The model under review builds one solid part; all positions refer to its coordinate system, in mm. A direction names the side the tool comes from. Give positions to 0.01 mm unless a question says otherwise; leave off trailing zeros. Order: outer loops, then holes, each group sorted by start corner. A loop starts at its lowest first (then second) coordinate and runs counter-clockwise, first axis right, second up. Notation, with made-up numbers: M 69.25,22 L 75.25,22 A19 ccw 75.25,54 Z; hole C 85.5,-0.75 d11. An arc over 180 degrees is marked long. One line per question, with ' | ' between items. Start each with the question number.
1. The part is to be moulded in two halves that separate along Y. For faces 1 (the face through (-73, 38, 0)), 2 (the face through (1, 60, 0)), 3 (the face through (-102, 1, 0)), say which applies: +Y half, -Y half, draft (parallel to the pull), parting line (faces both ways), or undercut.
2. We need section A-A on x = -76. Write out the cut boundary in (y, z), then the cut area to 4 significant figures.
3. We need section C-C on z = -1.75. Write out the cut boundary in (x, y).
4. We need section B-B on y = 34. Write out the cut boundary in (x, z).
5. Insertion check: P1, Ø4, axis at x = -96.5, y = -53, coming from the -Z side. The pin has a flat end and moves straight along its axis. Give the tip position at first contact, or say it passes through.
6. For faces 4 (the face through (-95.867, 49.095, -2.535)), 5 (the face through (75.9, 42.5, -2.5)), 6 (the face through (76, 45, 2)), 7 (the face through (-1, 1, -5)), list the 3-axis set-ups (+Z, -Z, +X, -X, +Y, -Y) from which the entire face can be reached by the end or side of a thin tool; tool diameter is ignored.
7. Wall thickness on L1, parallel to X at y = 36, z = 4; L2, parallel to Y at x = -95, z = -2.1; L3, parallel to Y at x = -95, z = 3: over which ranges is each line inside the solid? List them lowest first.
```python
from build123d import *

# Parameters (mm, degrees)
F0_R     = 4
F1_DEPTH = 5
F2_DEPTH = 5
F3_DEPTH = 5
F0_R_2   = 1.6
F4_DEPTH = 5
F5_DEPTH = 5
F6_DEPTH = 5
F7_DEPTH = 5
F8_DEPTH = 5


with BuildPart() as f1:
    # F0 (on Top) → F1 (new body)
    with BuildSketch(Plane.XY):
        Polygon((102, 53), (102, 60), (95, 60), (-95, 60), (-102, 60), (-102, 53), (-102, -53), (-102, -60), (-95, -60), (95, -60), (102, -60), (102, -53), align=None)
        with Locations((-95, -53)):
            Circle(F0_R, mode=Mode.SUBTRACT)
        with Locations((95, -53)):
            Circle(F0_R, mode=Mode.SUBTRACT)
        with BuildLine():
            ThreePointArc((-81, 40), (-76, 45), (-71, 40))
            Line((-71, 40), (-71, 27))
            ThreePointArc((-71, 27), (-76, 22), (-81, 27))
            Line((-81, 27), (-81, 40))
        make_face(mode=Mode.SUBTRACT)
        with Locations((-95, 53)):
            Circle(F0_R, mode=Mode.SUBTRACT)
        with BuildLine():
            Line((71, 27), (71, 40))
            ThreePointArc((71, 40), (76, 45), (81, 40))
            Line((81, 40), (81, 27))
            ThreePointArc((81, 27), (76, 22), (71, 27))
        make_face(mode=Mode.SUBTRACT)
        with Locations((95, 53)):
            Circle(F0_R, mode=Mode.SUBTRACT)
    extrude(amount=-F1_DEPTH)

    # F0 (on Top) → F2 (join)
    with BuildSketch(Plane.XY):
        with BuildLine():
            Line((-71, 27), (-71, 40))
            ThreePointArc((-71, 40), (-76, 45), (-81, 40))
            Line((-81, 40), (-81, 27))
            ThreePointArc((-81, 27), (-80.330127, 29.5), (-78.5, 31.330127))
            Line((-78.5, 31.330127), (-78.5, 40))
            ThreePointArc((-78.5, 40), (-76, 42.5), (-73.5, 40))
            Line((-73.5, 40), (-73.5, 31.330127))
            ThreePointArc((-73.5, 31.330127), (-71.669873, 29.5), (-71, 27))
        make_face()
    extrude(amount=-F2_DEPTH)

    # F0 (on Top) → F3 (join)
    with BuildSketch(Plane.XY):
        Polygon((102, 53), (102, 60), (95, 60), (-95, 60), (-102, 60), (-102, 53), (-102, -53), (-102, -60), (-95, -60), (95, -60), (102, -60), (102, -53), align=None)
        with Locations((-95, -53)):
            Circle(F0_R, mode=Mode.SUBTRACT)
        with Locations((95, -53)):
            Circle(F0_R, mode=Mode.SUBTRACT)
        with BuildLine():
            ThreePointArc((-81, 40), (-76, 45), (-71, 40))
            Line((-71, 40), (-71, 27))
            ThreePointArc((-71, 27), (-76, 22), (-81, 27))
            Line((-81, 27), (-81, 40))
        make_face(mode=Mode.SUBTRACT)
        with Locations((-95, 53)):
            Circle(F0_R, mode=Mode.SUBTRACT)
        with BuildLine():
            Line((71, 27), (71, 40))
            ThreePointArc((71, 40), (76, 45), (81, 40))
            Line((81, 40), (81, 27))
            ThreePointArc((81, 27), (76, 22), (71, 27))
        make_face(mode=Mode.SUBTRACT)
        with Locations((95, 53)):
            Circle(F0_R, mode=Mode.SUBTRACT)
    extrude(amount=F3_DEPTH)

    # F0 (on Top) → F4 (join)
    with BuildSketch(Plane.XY):
        with Locations((95, -53)):
            Circle(F0_R)
        with Locations((95, -53)):
            Circle(F0_R_2, mode=Mode.SUBTRACT)
    extrude(amount=F4_DEPTH)

    # F0 (on Top) → F5 (join)
    with BuildSketch(Plane.XY):
        with BuildLine():
            ThreePointArc((81, 40), (76, 45), (71, 40))
            Line((71, 40), (71, 27))
            ThreePointArc((71, 27), (71.669873, 29.5), (73.5, 31.330127))
            Line((73.5, 31.330127), (73.5, 40))
            ThreePointArc((73.5, 40), (76, 42.5), (78.5, 40))
            Line((78.5, 40), (78.5, 31.330127))
            ThreePointArc((78.5, 31.330127), (80.330127, 29.5), (81, 27))
            Line((81, 27), (81, 40))
        make_face()
    extrude(amount=-F5_DEPTH)

    # F0 (on Top) → F6 (join)
    with BuildSketch(Plane.XY):
        with Locations((95, 53)):
            Circle(F0_R)
        with Locations((95, 53)):
            Circle(F0_R_2, mode=Mode.SUBTRACT)
    extrude(amount=F6_DEPTH)

    # F0 (on Top) → F7 (join)
    with BuildSketch(Plane.XY):
        with Locations((-95, 53)):
            Circle(F0_R)
        with Locations((-95, 53)):
            Circle(F0_R_2, mode=Mode.SUBTRACT)
    extrude(amount=F7_DEPTH)

    # F0 (on Top) → F8 (join)
    with BuildSketch(Plane.XY):
        with Locations((-95, -53)):
            Circle(F0_R)
        with Locations((-95, -53)):
            Circle(F0_R_2, mode=Mode.SUBTRACT)
    extrude(amount=F8_DEPTH)


solid = f1.part
```
Entries:
1) face 1: undercut | face 2: +Y half | face 3: draft
2) outline: M -60,-5 L 22,-5 L 22,5 L -60,5 Z; M 42.5,-5 L 60,-5 L 60,5 L 45,5 L 45,0 L 42.5,0 Z | area: 982.5 mm^2
3) outline: M -102,-60 L 102,-60 L 102,60 L -102,60 Z; hole C -95,-53 d8; hole C -95,53 d8; hole M -78.5,31.33 A5 ccw long -73.5,31.33 L -73.5,40 A2.5 ccw -78.5,40 Z; hole M 73.5,31.33 A5 ccw long 78.5,31.33 L 78.5,40 A2.5 ccw 73.5,40 Z; hole C 95,-53 d8; hole C 95,53 d8
4) outline: M -102,-5 L -78.5,-5 L -78.5,0 L -81,0 L -81,5 L -102,5 Z; M -73.5,-5 L 73.5,-5 L 73.5,0 L 71,0 L 71,5 L -71,5 L -71,0 L -73.5,0 Z; M 78.5,-5 L 102,-5 L 102,5 L 81,5 L 81,0 L 78.5,0 Z
5) P1: stops at z = 0
6) face 4: -Z | face 5: +Z, -Z | face 6: +Z | face 7: -Z, +X, -X, +Y, -Y
7) L1: x = -102 to -81, -71 to 71, 81 to 102 | L2: y = -60 to -57, -49 to 49, 57 to 60 | L3: y = -60 to -54.6, -51.4 to 51.4, 54.6 to 60
